Design review of the part built by this model. Coordinates are the model's own, in mm. Coordinates: 2 decimals unless noted, no trailing zeros. Loops run counter-clockwise (first coordinate to the right, second up) from the corner with the lowest first, then second, coordinate; pieces in that order, holes last. Notation, with made-up numbers: (-35, 19.5) -> (-14, 19.5) arc R33 cw to (-14, 57.5) -> close; hole circle Ø8 at (-4, -17.75). An arc over 180 degrees is marked (long way). Use a Markdown table: item, result. Add a question column.
Q1. Take a section at B-B on x = 0. Write out the cut boundary in (y, z), plus the area to 3 significant figures.
Q2. Take a section at C-C on x = 72.5. Write out the cut boundary in (y, z), plus the area to 3 significant figures.
Q3. Take a section at A-A on z = 2.55. Write out the cut boundary in (x, y), plus the area to 3 significant figures.
Q4. Clearance check with flat-ended pins moving along their axes: pin 1 Ø0.9 at (x, z) = (87, 2) entering from -Y; pin 2 Ø0.9 at (x, z) = (4.5, 1) entering from -Y; pin 3 Ø1.5 at (x, z) = (31, 2) entering from -Y. State where each tip first meets the part, or that it passes through.
Q5. For probe 1 along X at (y, z) = (0, 2.2); probe 2 along X at (y, z) = (2.3, 2.7); probe 3 along X at (y, z) = (0.9, 1.15), list the stretches that pass through material, from the lowest coordinate up.
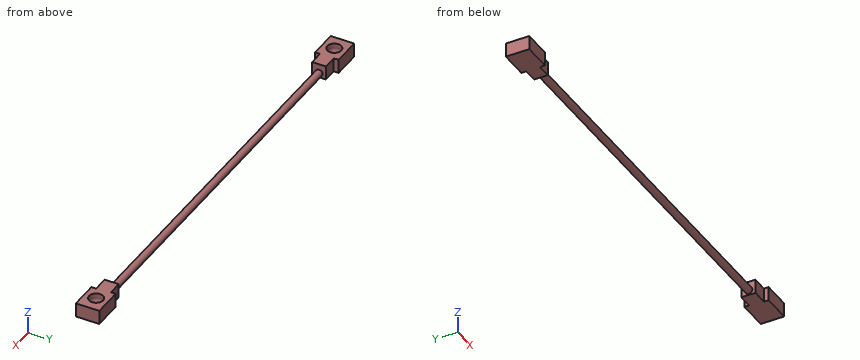
from build123d import *

# Parameters (mm, degrees)
BOSS_EXTRUDE1_DEPTH = 3
SKETCH2_R           = 1.5
CUT_EXTRUDE1_DEPTH  = 1
SKETCH3_R           = 0.75
BOSS_EXTRUDE2_DEPTH = 80
BOSS_EXTRUDE3_DEPTH = 3
SKETCH7_R           = 1.5
CUT_EXTRUDE2_DEPTH  = 1


with BuildPart() as part:
    # Sketch1 → Boss-Extrude1 (new body)
    with BuildSketch(Plane.XY):
        Polygon((-3.106795218, -2.5), (-3.106795218, 2.5), (2.893204782, 2.5), (2.893204782, 1.464436404), (5.893204782, 1.464436404), (5.893204782, -1.464436404), (2.893204782, -1.464436404), (2.893204782, -2.5), align=None)
    extrude(amount=BOSS_EXTRUDE1_DEPTH)

    # Sketch2 → Cut-Extrude1 (cut)
    with BuildSketch(Plane.XY.offset(3)):
        Circle(SKETCH2_R)
    extrude(amount=-CUT_EXTRUDE1_DEPTH, mode=Mode.SUBTRACT)

    # Sketch3 → Boss-Extrude2 (add)
    with BuildSketch(Plane(origin=(5.893204782, 0, 0), x_dir=(0, 0, -1), z_dir=(1, 0, 0))):
        with Locations(Location((-1, 0, 0), (0, 0, 180))):
            Circle(SKETCH3_R)
    extrude(amount=BOSS_EXTRUDE2_DEPTH)

    # Sketch4 → Boss-Extrude3 (add)
    with BuildSketch(Plane.XY):
        Polygon((85.893204782, 0.75), (85.893204782, 1.606881618), (88.893204782, 1.606881618), (88.893204782, 2.606881618), (95.170891527, 2.606881618), (95.170891527, -2.393118382), (89.170891527, -2.393118382), (89.170891527, -1.393118382), (85.893204782, -1.393118382), (85.893204782, -0.75), align=None)
    extrude(amount=BOSS_EXTRUDE3_DEPTH)

    # Sketch7 → Cut-Extrude2 (cut)
    with BuildSketch(Plane.XY.offset(3)):
        with Locations((91.865552177, 0.106881618)):
            Circle(SKETCH7_R)
    extrude(amount=-CUT_EXTRUDE2_DEPTH, mode=Mode.SUBTRACT)

    # Sketch8 → Cut-Revolve1 (revolve, cut)
    with BuildSketch(Plane.XY.offset(2)):
        with BuildLine():
            Line((91.865552177, 1.606881618), (91.865552177, -1.393118382))
            ThreePointArc((91.865552177, -1.393118382), (93.365552177, 0.106881618), (91.865552177, 1.606881618))
        make_face()
    revolve(axis=Axis((91.865552177, -999.893118382, 2), (0, 1, 0)), mode=Mode.SUBTRACT)

    # Sketch9 → Cut-Revolve2 (revolve, cut)
    with BuildSketch(Plane.XY.offset(2)):
        with BuildLine():
            Line((0, 1.5), (0, -1.5))
            ThreePointArc((0, -1.5), (1.5, 0), (0, 1.5))
        make_face()
    revolve(axis=Axis((0, -1000, 2), (0, 1, 0)), mode=Mode.SUBTRACT)


solid = part.part
Answer list:
| question | item | result |
|---|---|---|
| 1 | outline | (-2.5, 0) -> (2.5, 0) -> (2.5, 3) -> (1.5, 3) -> (1.5, 2) arc R1.5 cw to (-1.5, 2) -> (-1.5, 3) -> (-2.5, 3) -> close |
| 1 | area | 8.47 mm² |
| 2 | outline | circle Ø1.5 at (0, 1) |
| 2 | area | 1.77 mm² |
| 3 | outline | (-3.11, -2.5) -> (2.89, -2.5) -> (2.89, -1.46) -> (5.89, -1.46) -> (5.89, 1.46) -> (2.89, 1.46) -> (2.89, 2.5) -> (-3.11, 2.5) -> close; (85.89, -1.39) -> (89.17, -1.39) -> (89.17, -2.39) -> (95.17, -2.39) -> (95.17, 2.61) -> (88.89, 2.61) -> (88.89, 1.61) -> (85.89, 1.61) -> close; hole circle Ø3 at (0, 0); hole circle Ø3 at (91.87, 0.11) |
| 3 | area | 64.8 mm² |
| 4 | pin 1 | y = -1.39 |
| 4 | pin 2 | y = -1.46 |
| 4 | pin 3 | y = -0.71 |
| 5 | probe 1 | -3.11 to -1.5, 1.5 to 5.89, 85.89 to 90.37, 93.36 to 95.17 |
| 5 | probe 2 | -3.11 to 2.89, 88.89 to 95.17 |
| 5 | probe 3 | -3.11 to -0.85, 0.85 to 5.89, 85.89 to 90.92, 92.81 to 95.17 |
